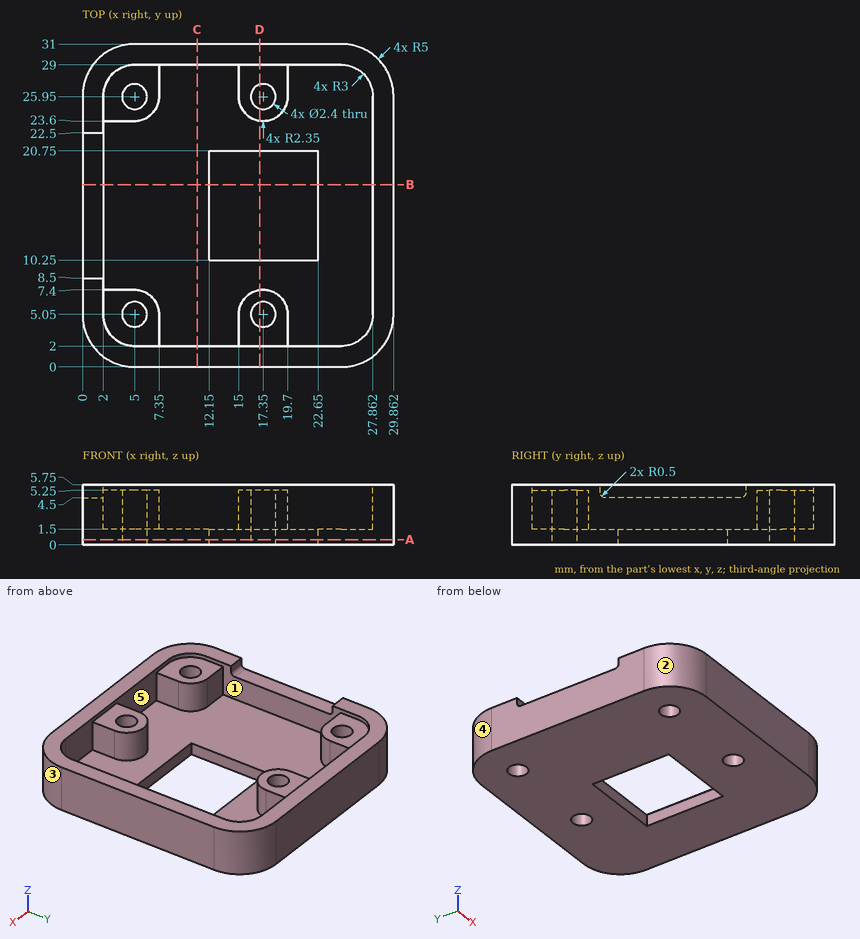
The figure shows three views and two pictorial views of one solid part (mm, origin at its lowest corner). Answer the questions. A direction names the side the tool comes from. Give positions to 0.01 mm unless a question says otherwise; leave off trailing zeros. Write each loop counter-clockwise with the first axis right and the second up, starting at its lowest first coordinate (ties: lowest second). Pieces come first, ordered by that corner, then holes. Notation, with made-up numbers: M 72,16.25 L 90,16.25 A12 cw 90,27.25 Z; hole C -11,24.25 d10. An arc over 180 degrees is marked long. One line per item, written item: value. Start each with the question number.
(1) Flat-ended cylindrical pins translate along their axes: pin 1 Ø0.9 at (y, z) = (27.5, 4.5) entering from -X; pin 2 Ø1.4 at (x, y) = (17, 27) entering from +Z; pin 3 Ø2.5 at (y, z) = (27.5, 4) entering from +X. Find the tip coordinate at first contact, or state that the pin passes through.
(2) Determine the mould class of the marked faces 3, 4 and 5 for opening direction Y: pulls with the +Y half, pulls with the -Y half, needs draft (parallel to the pull), parting line crosses it, or undercut.
(3) Find the intervals of material crossed by line 1 (Y direction, x = 17.35, z = 1.15); line 2 (Y direction, x = 17.35, z = 1.95); line 3 (Y direction, x = 11, z = 1.85), in increasing order.
(4) Find section D-D (x = 17). Determine the outline of the cut face in (y, z), plus the area to 3 significant figures.
(5) A tool of negligible diameter and unlimited length cuts with its end or side. For the marked faces 1 and 2, from which of +Z, -Z, +X, -X, +Y, -Y can it reach the whole face along a straight path? Write none if from no direction.
(6) Find section A-A (z = 0.5). Determine the outline of the cut face in (x, y).
(7) Find section B-B (y = 17.5). Determine the outline of the cut face in (x, z), plus the area to 3 significant figures.
(8) Find section C-C (x = 11). Determine the outline of the cut face in (y, z).
Results below:
1. pin 1: stops at x = 0.11
1. pin 2: stops at z = 5.25
1. pin 3: stops at x = 29.86
2. face 3: pulls with the -Y half
2. face 4: pulls with the +Y half
2. face 5: undercut
3. line 1: y = 0 to 3.85, 6.25 to 10.25, 20.75 to 24.75, 27.15 to 31
3. line 2: y = 0 to 3.85, 6.25 to 7.4, 23.6 to 24.75, 27.15 to 31
3. line 3: y = 0 to 2, 29 to 31
4. outline: M 0,0 L 3.9,0 L 3.9,5.25 L 2,5.25 L 2,5.75 L 0,5.75 Z; M 6.2,0 L 10.25,0 L 10.25,1.5 L 7.37,1.5 L 7.37,5.25 L 6.2,5.25 Z; M 20.75,0 L 24.8,0 L 24.8,5.25 L 23.63,5.25 L 23.63,1.5 L 20.75,1.5 Z; M 27.1,0 L 31,0 L 31,5.75 L 29,5.75 L 29,5.25 L 27.1,5.25 Z
4. area: 63.9 mm^2
5. face 1: +Z
5. face 2: +Z, -Z, -X, -Y
6. outline: M 0,5 A5 ccw 5,0 L 24.86,0 A5 ccw 29.86,5 L 29.86,26 A5 ccw 24.86,31 L 5,31 A5 ccw 0,26 Z; hole C 5,5.05 d2.4; hole C 5,25.95 d2.4; hole M 12.15,10.25 L 22.65,10.25 L 22.65,20.75 L 12.15,20.75 Z; hole C 17.35,5.05 d2.4; hole C 17.35,25.95 d2.4
7. outline: M 0,0 L 12.15,0 L 12.15,1.5 L 2,1.5 L 2,4.5 L 0,4.5 Z; M 22.65,0 L 29.86,0 L 29.86,5.75 L 27.86,5.75 L 27.86,1.5 L 22.65,1.5 Z
7. area: 43.5 mm^2
8. outline: M 0,0 L 31,0 L 31,5.75 L 29,5.75 L 29,1.5 L 2,1.5 L 2,5.75 L 0,5.75 Z
